Verification items for the finished model (mm, model axes). A direction names the side the tool comes from. Coordinates: 2 decimals unless noted, no trailing zeros. Write each loop counter-clockwise with the first axis right and the second up, starting at its lowest first coordinate (ties: lowest second). Pieces come first, ordered by that corner, then holes. Notation, with made-up numbers: (89, 23) - (139, 23) arc R9 ccw to (139, 32) - close; hole circle Ø8 at (72.5, -32). An arc over 180 degrees is marked (long way). Answer as CSV lines item,"result". Start each with the question number.
```python
from build123d import *

# Parameters (mm, degrees)
SKETCH_1_R          = 1.5
SKETCH_1_R_2        = 4.5
SKETCH_1_R_3        = 2.096788488
SKETCH_1_R_4        = 2
SKETCH_1_W          = 4.4
SKETCH_1_H          = 8.4
EXTRUDE_1_DEPTH     = 4
SKETCH_2_R          = 2
CUT_EXTRUDE_1_DEPTH = 10


with BuildPart() as part:
    # 草图1 → 凸台-拉伸1 (new body)
    with BuildSketch(Plane.XY):
        Polygon((-6, 39), (134, 39), (134, -39), (-6, -39), (-80, -39), (-80, 39), align=None)
        Circle(SKETCH_1_R, mode=Mode.SUBTRACT)
        with Locations(Location((0, 26, 0), (0, 0, 180))):
            Circle(SKETCH_1_R, mode=Mode.SUBTRACT)
        with Locations((0, -26)):
            Circle(SKETCH_1_R, mode=Mode.SUBTRACT)
        with Locations((50, 0)):
            Circle(SKETCH_1_R_2, mode=Mode.SUBTRACT)
        with Locations((50, 20)):
            Circle(SKETCH_1_R_3, mode=Mode.SUBTRACT)
        with Locations((50, -20)):
            Circle(SKETCH_1_R_3, mode=Mode.SUBTRACT)
        with Locations((90, -20)):
            Circle(SKETCH_1_R_3, mode=Mode.SUBTRACT)
        with Locations((90, 20)):
            Circle(SKETCH_1_R_3, mode=Mode.SUBTRACT)
        with Locations((10, -20)):
            Circle(SKETCH_1_R_4, mode=Mode.SUBTRACT)
        with Locations(Location((10, 20, 0), (0, 0, 180))):
            Circle(SKETCH_1_R_4, mode=Mode.SUBTRACT)
        with Locations(Location((-74, 0, 0), (0, 0, 180))):
            Circle(SKETCH_1_R, mode=Mode.SUBTRACT)
        with Locations((-74, 26)):
            Circle(SKETCH_1_R, mode=Mode.SUBTRACT)
        with Locations(Location((-74, -26, 0), (0, 0, 180))):
            Circle(SKETCH_1_R, mode=Mode.SUBTRACT)
        with Locations((0, 13)):
            Rectangle(SKETCH_1_W, SKETCH_1_H, mode=Mode.SUBTRACT)
        with Locations((0, -13)):
            Rectangle(SKETCH_1_W, SKETCH_1_H, mode=Mode.SUBTRACT)
        with Locations((-74, 13)):
            Rectangle(SKETCH_1_W, SKETCH_1_H, mode=Mode.SUBTRACT)
        with Locations((-74, -13)):
            Rectangle(SKETCH_1_W, SKETCH_1_H, mode=Mode.SUBTRACT)
    extrude(amount=EXTRUDE_1_DEPTH)

    # 草图2 → 切除-拉伸1 (cut)
    with BuildSketch(Plane(origin=(0, 0, 0), x_dir=(-1, 0, 0), z_dir=(0, 0, -1))):
        with Locations((-128, -33)):
            Circle(SKETCH_2_R)
        with Locations((-48, -33)):
            Circle(SKETCH_2_R)
        with Locations((-48, 33)):
            Circle(SKETCH_2_R)
        with Locations((-128, 33)):
            Circle(SKETCH_2_R)
        Polygon((61.8, -12.773298845), (24.525364108, 29), (61.8, 29), align=None)
        Polygon((12.2, -29), (49.474635892, -29), (12.2, 12.773298845), align=None)
    extrude(amount=-CUT_EXTRUDE_1_DEPTH, mode=Mode.SUBTRACT)


solid = part.part
```
1. Draft check along X on faces 1 (the face through (26, -39, 2)), 2 (the face through (-80, -1, 2)), 3 (the face through (48, 31, 2)). Enter one of: pulls with the +X half, pulls with the -X half, needs draft (parallel to the pull), parting line crosses it, or undercut.
2. Cross-section at A-A (x = 10). Record the cut outline in (y, z).
3. Scan lines: line 1 along Y through (x, z) = (0, 3.15); line 2 along Y through (x, z) = (10, 2.75); line 3 along Y through (x, z) = (90, 1.6). Record each from-to range of solid material in increasing order. Write a range as from..to.
4. Cross-section at D-D (x = -52). Record the cut outline in (y, z), and give its area (3 significant figures).
5. Cross-section at B-B (y = 33). Record the cut outline in (x, z).
6. Access from +Z, -Z, +X, -X, +Y, -Y to the whole of each face (thin tool, end or side, straight path). Record for faces 4 (the face through (-31.1, -8.41, 1.97)), 5 (the face through (28, 1, 4)).
7. Cross-section at C-C (y = 20). Record the cut outline in (x, z), and give its area (3 significant figures).
Completed:
1,face 1,"needs draft"
1,face 2,"pulls with the -X half"
1,face 3,"undercut"
2,outline,"(-39, 0) - (-22, 0) - (-22, 4) - (-39, 4) - close; (-18, 0) - (18, 0) - (18, 4) - (-18, 4) - close; (22, 0) - (39, 0) - (39, 4) - (22, 4) - close"
3,line 1,"y = -39..-27.5, -24.5..-17.2, -8.8..-1.5, 1.5..8.8, 17.2..24.5, 27.5..39"
3,line 2,"y = -39..-22, -18..18, 22..39"
3,line 3,"y = -39..-22.1, -17.9..17.9, 22.1..39"
4,outline,"(-39, 0) - (-1.79, 0) - (-1.79, 4) - (-39, 4) - close; (29, 0) - (39, 0) - (39, 4) - (29, 4) - close"
4,area,"189 mm2"
5,outline,"(-80, 0) - (46, 0) - (46, 4) - (-80, 4) - close; (50, 0) - (126, 0) - (126, 4) - (50, 4) - close; (130, 0) - (134, 0) - (134, 4) - (130, 4) - close"
6,face 4,"+Z, -Z"
6,face 5,"+Z, +X, -X, +Y, -Y"
7,outline,"(-80, 0) - (-61.8, 0) - (-61.8, 4) - (-80, 4) - close; (-32.56, 0) - (8, 0) - (8, 4) - (-32.56, 4) - close; (12, 0) - (47.9, 0) - (47.9, 4) - (12, 4) - close; (52.1, 0) - (87.9, 0) - (87.9, 4) - (52.1, 4) - close; (92.1, 0) - (134, 0) - (134, 4) - (92.1, 4) - close"
7,area,"689 mm2"
